```python
from build123d import *

# Parameters (mm, degrees)
SKETCH1_W              = 2.7
SKETCH1_H              = 1.1
BOSS_EXTRUDE1_DEPTH    = 4
SKETCH2_W              = 2.7
SKETCH2_H              = 0.9
BOSS_EXTRUDE2_DEPTH    = 4
SKETCH3_W              = 2.7
SKETCH3_H              = 1.1
LENGHT_EXTRUSION_DEPTH = 125
BOSS_EXTRUDE4_DEPTH    = 1
FILLET8_R              = 0.5
SKETCH7_R              = 0.45
CUT_EXTRUDE1_DEPTH     = 0.9


with BuildPart() as part:
    # Sketch1 → Boss-Extrude1 (new body)
    with BuildSketch(Plane(origin=(0, 0, 0), x_dir=(1, 0, 0), z_dir=(0, 1, 0))):
        Rectangle(SKETCH1_W, SKETCH1_H)
    extrude(amount=BOSS_EXTRUDE1_DEPTH)

    # Sketch2 → Boss-Extrude2 (add)
    with BuildSketch(Plane(origin=(0, 4, 0), x_dir=(1, 0, 0), z_dir=(0, 1, 0))):
        with Locations((0, 0.1)):
            Rectangle(SKETCH2_W, SKETCH2_H)
    extrude(amount=BOSS_EXTRUDE2_DEPTH)

    # Sketch3 → lenght extrusion (add)
    with BuildSketch(Plane.XZ):
        with BuildLine():
            ThreePointArc((4, 3.215302113), (-2.302172887, 6.486387559), (-1.35, -0.55))
            Line((-1.35, -0.55), (-1.35, 0.55))
            Line((-1.35, 0.55), (1.35, 0.55))
            Line((1.35, 0.55), (1.35, -0.55))
            ThreePointArc((1.35, -0.55), (3.271085447, 0.913129226), (4, 3.215302113))
        make_face()
        Rectangle(SKETCH3_W, SKETCH3_H)
    extrude(amount=LENGHT_EXTRUSION_DEPTH)

    # Sketch6 → Boss-Extrude4 (add, symmetric)
    with BuildSketch(Plane(origin=(0, 0, 0), x_dir=(0, 0, -1), z_dir=(1, 0, 0))):
        Polygon((-0.55, 2.309401077), (-4.55, 0), (-0.55, 0), align=None)
    extrude(amount=BOSS_EXTRUDE4_DEPTH, both=True)

    # Fillet8
    # the kernel refuses this fillet: 0.5 mm, written as the material it adds along each edge
    with BuildSketch(Plane(origin=(-1.35, 0, 0.55), x_dir=(0, 1, 0), z_dir=(0, 0, -1))) as fillet8_piece_1_section:
        with BuildLine():
            CenterArc((FILLET8_R, -FILLET8_R), FILLET8_R, 90, 90)
            Line((0, -FILLET8_R), (0, 0))
            Line((0, 0), (FILLET8_R, 0))
        make_face()
    fillet8_piece_1 = extrude(amount=1.1, mode=Mode.PRIVATE)
    fillet8_piece_1 = fillet8_piece_1 & Plane(origin=(0, 0.115807934, 3.215302113), x_dir=(1, 0, 0), z_dir=(0, 1, 0)) * Cylinder(4, 5, mode=Mode.PRIVATE)
    add(fillet8_piece_1)
    with BuildSketch(Plane(origin=(1.35, 0, -0.55), x_dir=(0, 1, 0), z_dir=(0, 0, 1))) as fillet8_piece_2_section:
        with BuildLine():
            CenterArc((FILLET8_R, -FILLET8_R), FILLET8_R, 90, 90)
            Line((0, -FILLET8_R), (0, 0))
            Line((0, 0), (FILLET8_R, 0))
        make_face()
    fillet8_piece_2 = extrude(amount=1.1, mode=Mode.PRIVATE)
    fillet8_piece_2 = fillet8_piece_2 & Plane(origin=(0, 0.11580798, 3.215302113), x_dir=(1, 0, 0), z_dir=(0, 1, 0)) * Cylinder(4, 5, mode=Mode.PRIVATE)
    add(fillet8_piece_2)

    # Sketch7 → Cut-Extrude1 (cut)
    with BuildSketch(Plane.XY.offset(0.35)):
        with Locations((0, 5)):
            Circle(SKETCH7_R)
        with Locations((0, 7)):
            Circle(SKETCH7_R)
    extrude(amount=-CUT_EXTRUDE1_DEPTH, mode=Mode.SUBTRACT)


solid = part.part
```
Geometry: final body of the model. Coordinates: model frame, mm. A direction names the side the tool comes from. Coordinates: 2 decimals unless noted, no trailing zeros. Order: outer loops, then holes, each group sorted by start corner. A loop starts at its lowest first (then second) coordinate and runs counter-clockwise, first axis right, second up. Notation, with made-up numbers: M 39,44.5 L 63,44.5 A15 cw 63,68.5 Z; hole C -20.75,61 d9. An arc over 180 degrees is marked long. Answer in a Markdown table with one row per item. Add a question column.
Q1. Line query: L1, parallel to Y at x = 0, z = -0.05; L2, parallel to X at y = -87.5, z = 2.75; L3, parallel to Z at x = 0.25, y = -69. Output: solid intervals per line, ascending.
Q2. Reachability of faces 1 (the flat face through (1, 1, 2)), 2 (the flat face through (-1, 1, 2)), 3 (the flat face through (0, 6, 0.35)), 4 (the flat face through (0, -125, 3)), 5 (the flat face through (0, 2.5, 0.55)) from +Z, -Z, +X, -X, +Y, -Y: full face, straight path, thin tool, end or side. Return the list, or none.
Q3. Contact query for flat-ended pins moving along their axis: P1, Ø1.8, axis at x = 0, y = 1, coming from the +Z side; P2, Ø0.9, axis at y = 6, z = 0, coming from the +X side; P3, Ø2.5, axis at y = 1.5, z = 2, coming from the +X side. Output: stop coordinate, or through.
Q4. Section query A-A on y = -25. Return the cut outline in (x, z).
Completed:
| question | item | result |
|---|---|---|
| 1 | L1 | y = -125 to 4.55, 5.45 to 6.55, 7.45 to 8 |
| 1 | L2 | x = -3.97 to 3.97 |
| 1 | L3 | z = -0.55 to 7.21 |
| 2 | face 1 | +Z, +X, +Y |
| 2 | face 2 | +Z, -X, +Y |
| 2 | face 3 | +Z, +X, -X, +Y |
| 2 | face 4 | +Z, -Z, +X, -X, -Y |
| 2 | face 5 | +Z, +Y |
| 3 | P1 | stops at z = 4.38 |
| 3 | P2 | stops at x = 1.35 |
| 3 | P3 | stops at x = 1 |
| 4 | outline | M -1.35,-0.55 L 1.35,-0.55 A4 ccw long Z |
